Here's the drawing with two shaded views (mm, measured from the low corner). I have some questions. Give positions to 0.01 mm unless a question says otherwise; leave off trailing zeros. Write each loop counter-clockwise with the first axis right and the second up, starting at its lowest first coordinate (ties: lowest second). Pieces come first, ordered by that corner, then holes. Notation, with made-up numbers: (42.25, 81) - (90.25, 81) arc R13 cw to (90.25, 87) - close; hole circle Ø7 at (-7.5, 82). An arc over 180 degrees is marked (long way). Write item = value, one per line.
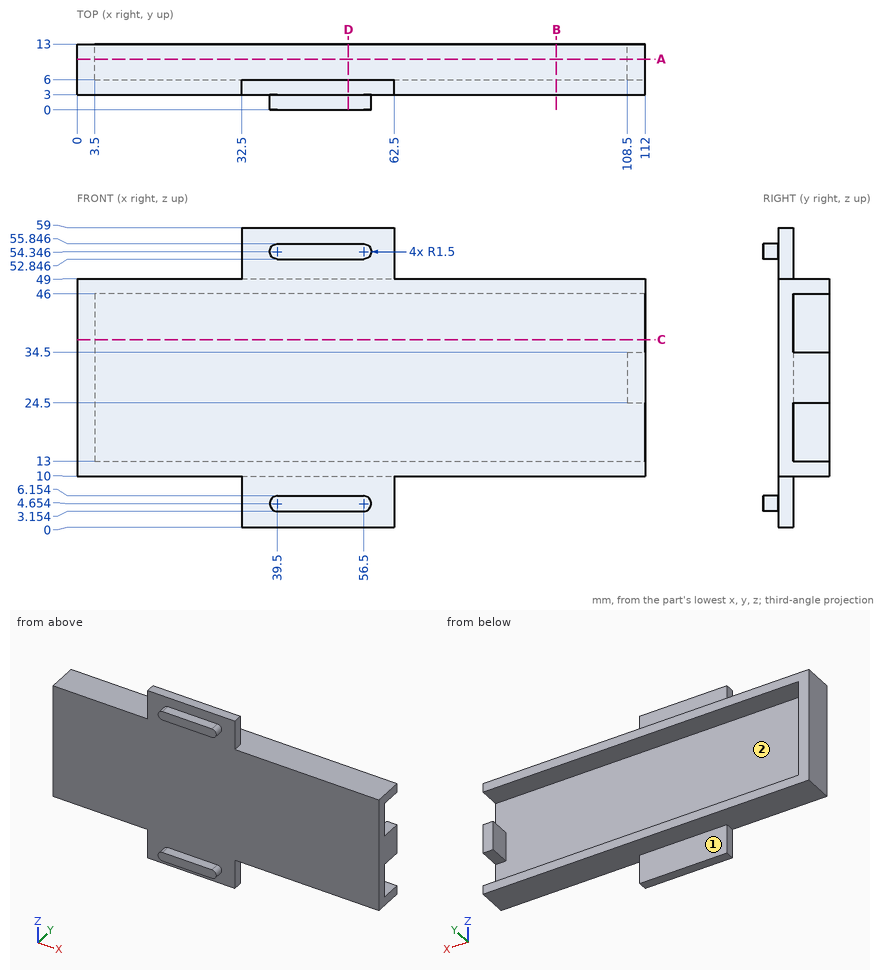
1. If we section it at C-C, the plane z = 37: Please give me the cut outline in (x, y), and give its area (4 significant figures).
Filled sheet:
outline = (0, 3) - (112, 3) - (112, 6) - (3.5, 6) - (3.5, 13) - (0, 13) - close
area = 360.5 mm2
2. If we section it at A-A, the plane y = 10: Please give me the cut outline in (x, z).
Filled sheet:
outline = (0, 10) - (112, 10) - (112, 13) - (3.5, 13) - (3.5, 46) - (112, 46) - (112, 49) - (0, 49) - close; (108.5, 24.5) - (112, 24.5) - (112, 34.5) - (108.5, 34.5) - close
3. Thinking about a two-plate mould opening in Z: for the marked faces 1 and 2, which applies, pulls with the +Z half, pulls with the -Z half, needs draft (parallel to the pull), parting line crosses it, or undercut?
Filled sheet:
face_1 = needs draft
face_2 = undercut
4. For pin 1 (2 mm diameter, centred on x = 54.5, y = 7.5, fed in from +Z); pin 2 (12 mm diameter, centred on x = 77, z = 37, fed in from +Y); pin 3 (2.5 mm diameter, centred on y = 5, z = 5, fed in from -X), each with a flat end and sliding along its axis, tell me the tip position at first contact or that it passes through.
Filled sheet:
pin_1 = 49
pin_2 = 6
pin_3 = 32.5
5. If we section it at D-D, the plane x = 53.5: Please give me the cut outline in (y, z), and give its area (3 significant figures).
Filled sheet:
outline = (0, 3.15) - (3, 3.15) - (3, 0) - (6, 0) - (6, 10) - (13, 10) - (13, 13) - (6, 13) - (6, 46) - (13, 46) - (13, 49) - (6, 49) - (6, 59) - (3, 59) - (3, 55.85) - (0, 55.85) - (0, 52.85) - (3, 52.85) - (3, 6.15) - (0, 6.15) - close
area = 237 mm2
6. If we section it at B-B, the plane x = 94.5: Please give me the cut outline in (y, z), and give its area (3 significant figures).
Filled sheet:
outline = (3, 10) - (13, 10) - (13, 13) - (6, 13) - (6, 46) - (13, 46) - (13, 49) - (3, 49) - close
area = 159 mm2
7. I need wall thicknesses on line 1 (Z direction, x = 86, y = 11.25); line 2 (Y direction, x = 37.5, z = 53); line 3 (Z direction, x = 50, y = 1.75). Which ranges of each line are inside material? Lowest first, please.
Filled sheet:
line_1 = 10 to 13, 46 to 49
line_2 = 3 to 6
line_3 = 3.15 to 6.15, 52.85 to 55.85
